```python
from build123d import *

# Parameters (mm, degrees)
BOSS_EXTRUDE1_DEPTH      = 5
TAP_DRILL_FOR_M10_TAP1_D = 8.5


with BuildPart() as part:
    # Sketch1 → Boss-Extrude1 (new body)
    with BuildSketch(Plane.XY):
        with BuildLine():
            Line((25, 0), (-25, 0))
            Line((-25, 0), (-25, 40))
            ThreePointArc((-25, 40), (-25.513167019, 43.16227766), (-27, 46))
            Line((-27, 46), (-33, 54))
            ThreePointArc((-33, 54), (-34.486832981, 56.83772234), (-35, 60))
            Line((-35, 60), (-35, 140))
            ThreePointArc((-35, 140), (-33.535533906, 143.535533906), (-30, 145))
            Line((-30, 145), (-17, 145))
            ThreePointArc((-17, 145), (-13.464466094, 143.535533906), (-12, 140))
            Line((-12, 140), (-12, 100))
            ThreePointArc((-12, 100), (0, 88), (12, 100))
            Line((12, 100), (12, 140))
            ThreePointArc((12, 140), (13.464466094, 143.535533906), (17, 145))
            Line((17, 145), (30, 145))
            ThreePointArc((30, 145), (33.535533906, 143.535533906), (35, 140))
            Line((35, 140), (35, 60))
            ThreePointArc((35, 60), (34.486832981, 56.83772234), (33, 54))
            Line((33, 54), (27, 46))
            ThreePointArc((27, 46), (25.513167019, 43.16227766), (25, 40))
            Line((25, 40), (25, 0))
        make_face()
    extrude(amount=BOSS_EXTRUDE1_DEPTH)

    # Tap Drill for M10 Tap1 (through all)
    with Locations(Plane.XY.offset(5)):
        with Locations((23.5, 130.17967031), (-23.5, 69.82032969)):
            Hole(TAP_DRILL_FOR_M10_TAP1_D / 2)


solid = part.part
```
Work out the finished part from the listing and answer in its coordinate system (mm). A direction names the side the tool comes from. Give positions to 0.01 mm unless a question says otherwise; leave off trailing zeros. Order: outer loops, then holes, each group sorted by start corner. A loop starts at its lowest first (then second) coordinate and runs counter-clockwise, first axis right, second up. Notation, with made-up numbers: M 6.5,-31.75 L 32.5,-31.75 A6 cw 32.5,-20.75 Z; hole C -8.75,-10 d8. An arc over 180 degrees is marked long. Return JSON: item names as keys, results as strings.
1) Section D-D, the plane x = 0 is taken. Write down the section's boundary in (y, z), plus the area to 3 significant figures.
Resolved:
{"outline": "M 0,0 L 88,0 L 88,5 L 0,5 Z", "area": "440 mm^2"}
2) For a pull along X with two mould halves and no side action, classify faces 1 (the cylindrical face through (13, 143, 2)), 2 (the cylindrical face through (-34.472, 56.795, 2.465)), 3 (the flat face through (23, 145, 2)), 4 (the flat face through (30, 50, 2)) as +X half, -X half, draft (parallel to the pull), parting line (faces both ways), or undercut.
Resolved:
{"face 1": "undercut", "face 2": "-X half", "face 3": "draft", "face 4": "+X half"}
3) Each of these flat-tipped pins is pushed along its axis until it touches: pin 1 (10 mm diameter, centred on x = 11, y = 89, fed in from -Z); pin 2 (7 mm diameter, centred on x = -23.5, y = 69.82, fed in from -Z); pin 3 (2.5 mm diameter, centred on y = 22, z = 3, fed in from +X). Where does it stop, or does it pass through?
Resolved:
{"pin 1": "z = 0", "pin 2": "through", "pin 3": "x = 25"}
4) Section B-B, the plane y = 98 is taken. Write down the section's boundary in (x, z).
Resolved:
{"outline": "M -35,0 L -11.83,0 L -11.83,5 L -35,5 Z; M 11.83,0 L 35,0 L 35,5 L 11.83,5 Z"}
5) Section A-A, the plane x = 23.5 is taken. Write down the section's boundary in (y, z).
Resolved:
{"outline": "M 0,0 L 125.93,0 L 125.93,5 L 0,5 Z; M 134.43,0 L 145,0 L 145,5 L 134.43,5 Z"}
6) A tool of negligible diameter and unlimited length cuts with its end or side. For faces 5 (the flat face through (25, 20, 2)), 6 (the flat face through (12, 120, 2)), 7 (the cylindrical face through (21.54, 126.41, 2.47)), 8 (the flat face through (-25, 20, 2)), from which of +Z, -Z, +X, -X, +Y, -Y can it reach the whole face along a straight path? Write none if from no direction.
Resolved:
{"face 5": "+Z, -Z, +X, -Y", "face 6": "+Z, -Z, +Y", "face 7": "+Z, -Z", "face 8": "+Z, -Z, -X, -Y"}
7) Straight lines are drawn through the part: line 1 along Y through (x, z) = (23.5, 3.2); line 2 along Y through (x, z) = (-24, 1.7); line 3 along X through (y, z) = (133, 1.3). For each, find the intervals that lie inside material, in ascending order. Write a range as [from, to].
Resolved:
{"line 1": "[0, 125.93], [134.43, 145]", "line 2": "[0, 65.6], [74.04, 145]", "line 3": "[-35, -12], [12, 20.32], [26.68, 35]"}
8) Section C-C, the plane z = 3 is taken. Write down the section's boundary in (x, y), plus the area to 3 significant figures.
Resolved:
{"outline": "M -35,60 A10 ccw -33,54 L -27,46 A10 cw -25,40 L -25,0 L 25,0 L 25,40 A10 cw 27,46 L 33,54 A10 ccw 35,60 L 35,140 A5 ccw 30,145 L 17,145 A5 ccw 12,140 L 12,100 A12 cw -12,100 L -12,140 A5 ccw -17,145 L -30,145 A5 ccw -35,140 Z; hole C -23.5,69.82 d8.5; hole C 23.5,130.18 d8.5", "area": "7,710 mm^2"}
